from build123d import *

# Parameters (mm, degrees)
SKETCH1_R           = 23.8125
EXTRUDE1_DEPTH      = 27.7368
EXTRUDE1_DEPTH_BACK = 85.852
CUT_EXTRUDE1_REACH  = 87.852
SKETCH2_R           = 23.8125
SKETCH2_R_2         = 18.8595
CUT_EXTRUDE3_START  = -27.7368
SKETCH4_R           = 28.575
CUT_EXTRUDE3_DEPTH  = 27.7368
SKETCH18_R          = 9.525
CUT_EXTRUDE4_DEPTH  = 0.254
SKETCH19_R          = 9.525
CUT_EXTRUDE5_DEPTH  = 0.254
CHAMFER1_SIZE       = 0.762
CIRPATTERN1_COUNT   = 4
SKETCH20_R          = 6.9469
EXTRUDE2_DEPTH      = 1.27


with BuildPart() as part:
    # Sketch1 → Extrude1 (new body, two sides)
    with BuildSketch(Plane(origin=(0, 0, 0), x_dir=(0, 0, -1), z_dir=(1, 0, 0))) as extrude1_sk:
        Circle(SKETCH1_R)
    extrude(amount=EXTRUDE1_DEPTH)
    extrude(extrude1_sk.sketch, amount=-EXTRUDE1_DEPTH_BACK)

    # Sketch2 → Cut-Extrude1 (cut, up to next)
    with BuildSketch(Plane(origin=(0, 0, 0), x_dir=(0, 0, -1), z_dir=(1, 0, 0)), mode=Mode.PRIVATE) as cut_extrude1_sk1:
        Circle(SKETCH2_R)
        with Locations((0, -4.191)):
            Circle(SKETCH2_R_2, mode=Mode.SUBTRACT)
    cut_extrude1_tool1 = extrude(cut_extrude1_sk1.sketch, amount=-CUT_EXTRUDE1_REACH, mode=Mode.PRIVATE) & part.part
    add(cut_extrude1_tool1.solids().sort_by_distance((0, 0, 23.138981))[0], mode=Mode.SUBTRACT)

    # Sketch4 → Cut-Extrude3 (cut)
    with BuildSketch(Plane.ZY.offset(CUT_EXTRUDE3_START)):
        Circle(SKETCH4_R)
        with BuildLine():
            Line((18.923, -14.455283714), (18.923, 14.465869871))
            Line((18.923, 14.465869871), (0, 27.715897117))
            Line((0, 27.715897117), (-18.923, 14.465869871))
            Line((-18.923, 14.465869871), (-18.923, -14.455283714))
            ThreePointArc((-18.923, -14.455283714), (0, -23.8125), (18.923, -14.455283714))
        make_face(mode=Mode.SUBTRACT)
    extrude(amount=CUT_EXTRUDE3_DEPTH, mode=Mode.SUBTRACT)

    # Sketch6 → Cut-Revolve2 (revolve, cut)
    with BuildSketch(Plane.XY, mode=Mode.PRIVATE) as cut_revolve2_sk:
        Polygon((4.713225965, 47.625), (27.7368, 7.747), (27.7368, 47.625), align=None)
    revolve(cut_revolve2_sk.sketch.rotate(Axis((3.612847264, -4.191, 0), (1, 0, 0)), 270), axis=Axis((3.612847264, -4.191, 0), (1, 0, 0)), mode=Mode.SUBTRACT)  # turned: the seam where the file's is

    # S2D0002 → Cut-Revolve3 (revolve, cut)
    with BuildSketch(Plane(origin=(9.652, 18.394824642, 12.869035589), x_dir=(0, 0.573576436, -0.819152044), z_dir=(1, 0, 0))):
        Polygon((0, 0), (6.1849, 0), (5.642306865, -2.5527), (4.9784, -3.216606865), (4.9784, -13.462), (0, -13.462), align=None)
    revolve(axis=Axis((9.652, 6.816028581, 4.761475303), (0, 0.819152044, 0.573576436)), mode=Mode.SUBTRACT)

    # Sketch8 → Cut-Revolve4 (revolve, cut)
    with BuildSketch(Plane(origin=(9.652, 18.394824642, -12.869035589), x_dir=(0, -0.573576436, -0.819152044), z_dir=(1, 0, 0))):
        Polygon((0, 0), (6.1849, 0), (5.642306865, -2.5527), (4.9784, -3.216606865), (4.9784, -13.462), (0, -13.462), align=None)
    revolve(axis=Axis((9.652, 6.816028581, -4.761475303), (0, 0.819152044, -0.573576436)), mode=Mode.SUBTRACT)

    # Sketch18 → Cut-Extrude4 (cut)
    with BuildSketch(Plane(origin=(0, 18.59764611, 13.022211999), x_dir=(1, 0, 0), z_dir=(0, 0.819152044, 0.573576436))):
        with Locations((9.652, 0.009141155)):
            Circle(SKETCH18_R)
    extrude(amount=-CUT_EXTRUDE4_DEPTH, mode=Mode.SUBTRACT)

    # Sketch19 → Cut-Extrude5 (cut)
    with BuildSketch(Plane(origin=(0, 18.59764611, -13.022211999), x_dir=(1, 0, 0), z_dir=(0, 0.819152044, -0.573576436))):
        with Locations((9.652, -0.009141155)):
            Circle(SKETCH19_R)
    extrude(amount=-CUT_EXTRUDE5_DEPTH, mode=Mode.SUBTRACT)

    # Sketch10 → Cut-Revolve6 (revolve, cut)
    with BuildSketch(Plane.XY, mode=Mode.PRIVATE) as cut_revolve6_sk:
        Polygon((0, 14.6685), (0, 13.716), (-3.81, 13.716), (-4.7625, 14.6685), align=None)
    revolve(cut_revolve6_sk.sketch.rotate(Axis((-5.000625, -4.191, 0), (1, 0, 0)), 90), axis=Axis((-5.000625, -4.191, 0), (1, 0, 0)), mode=Mode.SUBTRACT)  # turned: the seam where the file's is

    # Sketch12 → Cut-Revolve8 (revolve, cut)
    with BuildSketch(Plane.XY, mode=Mode.PRIVATE) as cut_revolve8_sk:
        Polygon((-85.852, 14.6685), (-85.852, 13.716), (-83.312, 13.716), (-82.3595, 14.6685), align=None)
    revolve(cut_revolve8_sk.sketch.rotate(Axis((-63.674625, -4.191, 0), (1, 0, 0)), 90), axis=Axis((-63.674625, -4.191, 0), (1, 0, 0)), mode=Mode.SUBTRACT)  # turned: the seam where the file's is

    # Chamfer1
    chamfer1_edges = [part.edges().sort_by_distance(p)[0] for p in [
        (-85.852, -4.191, -17.907),
    ]]
    chamfer(chamfer1_edges, length=CHAMFER1_SIZE)

    # Sketch13 → Revolve1 (revolve)
    with BuildSketch(Plane(origin=(0, 0, 0), x_dir=(0, -1, 0), z_dir=(0, 0, 1)), mode=Mode.PRIVATE) as revolve1_sk:
        with BuildLine():
            Line((4.191, 27.7368), (4.191, 59.7662))
            Line((4.191, 59.7662), (11.1125, 59.7662))
            ThreePointArc((11.1125, 59.7662), (11.83092049, 59.46862049), (12.1285, 58.7502))
            Line((12.1285, 58.7502), (12.1285, 27.7368))
            Line((12.1285, 27.7368), (4.191, 27.7368))
        make_face()
    revolve(revolve1_sk.sketch.rotate(Axis((26.44521, -4.191, 0), (1, 0, 0)), 270), axis=Axis((26.44521, -4.191, 0), (1, 0, 0)))  # turned: the seam where the file's is

    # S2D0001 → Cut-Revolve9 (revolve, cut)
    with BuildSketch(Plane(origin=(54.6354, -8.4074, 0), x_dir=(0, -1, 0), z_dir=(0, 0, 1)), mode=Mode.PRIVATE) as cut_revolve9_sk:
        Polygon((0, 5.1308), (0, -10.1092), (-4.2164, -12.642668714), (-4.2164, 5.1308), align=None)
    revolve(cut_revolve9_sk.sketch.rotate(Axis((35.97325785, -4.191, 0), (1, 0, 0)), 270), axis=Axis((35.97325785, -4.191, 0), (1, 0, 0)), mode=Mode.SUBTRACT)  # turned: the seam where the file's is

    # Sketch16 → Cut-Revolve10 (revolve, cut)
    with BuildSketch(Plane(origin=(50.673, 1.421660076, -5.612660076), x_dir=(-1, 0, 0), z_dir=(0, -0.707106781, -0.707106781)), mode=Mode.PRIVATE) as cut_revolve10_sk:
        Polygon((-5.1308, 0), (-2.7178, 0), (-5.1308, -2.413), align=None)
    cut_revolve10 = revolve(cut_revolve10_sk.sketch.rotate(Axis((55.8038, -2.1640922, -2.0269078), (0, 0.707106781, -0.707106781)), 90), axis=Axis((55.8038, -2.1640922, -2.0269078), (0, 0.707106781, -0.707106781)), mode=Mode.SUBTRACT)  # turned: the seam where the file's is

    # CirPattern1: Cut-Revolve10 ×4 about axis
    cirpattern1_axis = Axis((26.44521, -4.191, 0), (-1, 0, 0))
    for i in range(1, CIRPATTERN1_COUNT):
        add(cut_revolve10.rotate(cirpattern1_axis, i * 360 / CIRPATTERN1_COUNT), mode=Mode.SUBTRACT)

    # Sketch20 → Extrude2 (add)
    with BuildSketch(Plane(origin=(0, 18.389581491, -12.876523585), x_dir=(1, 0, 0), z_dir=(0, 0.819152044, -0.573576436))):
        with Locations(Location((9.652, -0.009141155, 0), (0, 0, 270))):  # turned: the seam where the file's is
            Circle(SKETCH20_R)
    extrude(amount=EXTRUDE2_DEPTH)

    # Sketch21 → Cut-Revolve11 (revolve, cut)
    with BuildSketch(Plane.XY, mode=Mode.PRIVATE) as cut_revolve11_sk:
        Polygon((-71.882, -4.191), (-85.852, -4.191), (-85.852, -10.3759), (-83.2866, -9.830607397), (-82.625392603, -9.1694), (-71.882, -9.1694), align=None)
    revolve(cut_revolve11_sk.sketch.rotate(Axis((-37.427759391, -4.191, 0), (-1, 0, 0)), 90), axis=Axis((-37.427759391, -4.191, 0), (-1, 0, 0)), mode=Mode.SUBTRACT)  # turned: the seam where the file's is


solid = part.part
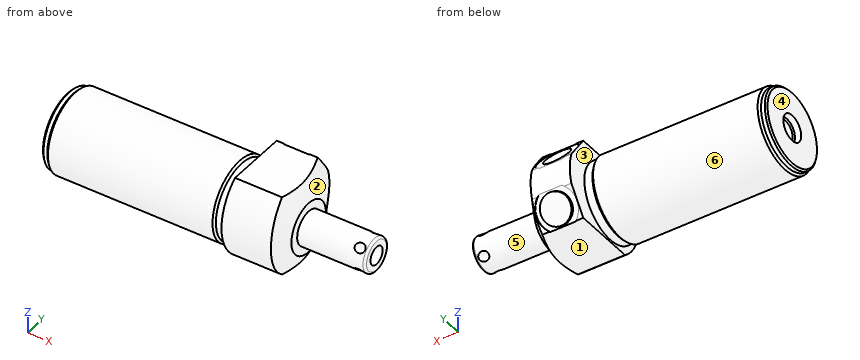
The listing builds one solid part. Answer for the finished solid, in the listing's coordinates (mm). Face numbers are marked on the shaded views. A direction names the side the tool comes from. Give positions to 0.01 mm unless a question says otherwise; leave off trailing zeros. Write each loop counter-clockwise with the first axis right and the second up, starting at its lowest first coordinate (ties: lowest second). Pieces come first, ordered by that corner, then holes. Notation, with made-up numbers: (84, -7) -> (134, -7) arc R16 cw to (134, 5) -> close; hole circle Ø11 at (-25.5, -38). An arc over 180 degrees is marked (long way). Use a Markdown table: item, result.
(1) Flat-ended cylindrical pins translate along their axes: P1, Ø3, axis at y = -3, z = 2.5, coming from the -X side; P2, Ø1.5, axis at x = -30, y = 10, coming from the +Z side; P3, Ø2, axis at y = -15.5, z = -14.5, coming from the +X side. Find the tip coordinate at first contact, or state that the pin passes through.
Return value:
| item | result |
|---|---|
| P1 | x = -71.88 |
| P2 | z = 13.23 |
| P3 | x = 24.59 |
(2) Determine the mould class of the marked faces 1, 2 and 3 for opening direction X: released by +X, released by -X, zero draft, split by the parting line, or undercut.
Return value:
| item | result |
|---|---|
| face 1 | zero draft |
| face 2 | released by +X |
| face 3 | undercut |
(3) Section A-A, the plane x = -17.5 is taken. Determine the outline of the cut face in (y, z), then the cut area to 3 significant figures.
Return value:
| item | result |
|---|---|
| outline | circle Ø37.72 at (-4.19, 0) |
| area | 1,120 mm2 |
(4) Find the intervals of material crossed by probe 1 along Y at (x, z) = (54, 0); probe 2 along Y at (x, z) = (-75.5, 0); probe 3 along X at (y, z) = (3, 8.5), in increasing order. Write a range as from..to.
Return value:
| item | result |
|---|---|
| probe 1 | -12.13..-8.41, 0.03..3.75 |
| probe 2 | -23.05..-9.17, 0.79..14.67 |
| probe 3 | -85.85..27.74 |
(5) For the marked faces 4, 5 and 6, determine the directions among +Z, -Z, +X, -X, +Y, -Y from which every point of the face is accessible in a straight line to the end or side of a thin tool.
Return value:
| item | result |
|---|---|
| face 4 | +Z, -Z, -X, +Y, -Y |
| face 5 | +X |
| face 6 | -X |
